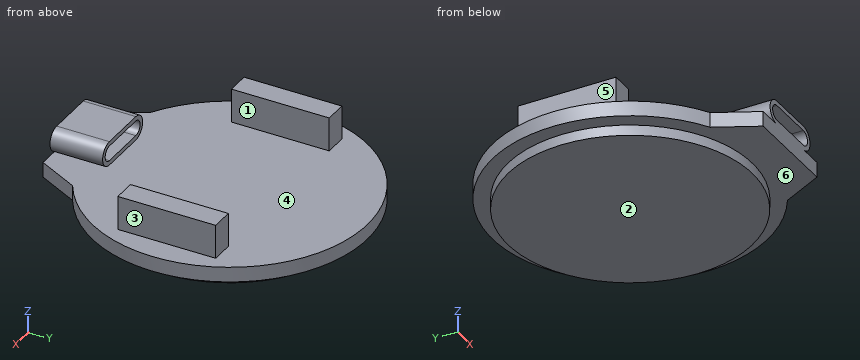
from build123d import *

# Parameters (mm, degrees)
EXTRUDE_1_DEPTH = 2
SKETCH_2_R      = 16.2
EXTRUDE_2_DEPTH = 1.4
SKETCH_3_W      = 3
SKETCH_3_H      = 13
EXTRUDE_3_DEPTH = 4.5
EXTRUDE_4_DEPTH = 7


with BuildPart() as part:
    # 草图1 → 凸台-拉伸1 (new body)
    with BuildSketch(Plane.XY):
        with BuildLine():
            Line((-6.405, -21.250170418), (6.405, -21.250170418))
            Line((6.405, -21.250170418), (9.185, -15.770170418))
            ThreePointArc((9.185, -15.770170418), (0, 18.25), (-9.185, -15.770170418))
            Line((-9.185, -15.770170418), (-6.405, -21.250170418))
        make_face()
    extrude(amount=EXTRUDE_1_DEPTH)

    # 草图2 → 凸台-拉伸2 (add)
    with BuildSketch(Plane(origin=(0, 0, 0), x_dir=(-1, 0, 0), z_dir=(0, 0, -1))):
        Circle(SKETCH_2_R)
    extrude(amount=EXTRUDE_2_DEPTH)

    # 草图3 → 凸台-拉伸3 (add)
    with BuildSketch(Plane.XY.offset(2)):
        with Locations((-13.5, 0)):
            Rectangle(SKETCH_3_W, SKETCH_3_H)
        with Locations((13.5, 0)):
            Rectangle(SKETCH_3_W, SKETCH_3_H)
    extrude(amount=EXTRUDE_3_DEPTH)

    # 草图4 → 凸台-拉伸4 (add)
    with BuildSketch(Plane.XZ.offset(21.250170418)):
        with BuildLine():
            Line((-3.15, 5.2), (3.15, 5.2))
            ThreePointArc((3.15, 5.2), (4.75, 3.6), (3.15, 2))
            Line((3.15, 2), (-3.15, 2))
            ThreePointArc((-3.15, 2), (-4.75, 3.6), (-3.15, 5.2))
        make_face()
        with BuildLine():
            Line((-3.15, 4.6), (3.15, 4.6))
            ThreePointArc((3.15, 4.6), (4.15, 3.6), (3.15, 2.6))
            Line((3.15, 2.6), (-3.15, 2.6))
            ThreePointArc((-3.15, 2.6), (-4.15, 3.6), (-3.15, 4.6))
        make_face(mode=Mode.SUBTRACT)
    extrude(amount=-EXTRUDE_4_DEPTH)


solid = part.part
The listing builds one solid part. Answer for the finished solid, in the listing's coordinates (mm). Face numbers are marked on the shaded views. A direction names the side the tool comes from. Coordinates: 2 decimals unless noted, no trailing zeros. Write each loop counter-clockwise with the first axis right and the second up, starting at its lowest first coordinate (ties: lowest second). Pieces come first, ordered by that corner, then holes. Notation, with made-up numbers: (-31, 79.5) -> (9, 79.5) arc R30 ccw to (9, 114.5) -> close; hole circle Ø11 at (-9, 67.5). An arc over 180 degrees is marked (long way). One line per question, with ' | ' between items.
1. Section A-A (x = 0) is taken. Determine the outline of the cut face in (y, z).
Verdict:
outline: (-21.25, 0) -> (-16.2, 0) -> (-16.2, -1.4) -> (16.2, -1.4) -> (16.2, 0) -> (18.25, 0) -> (18.25, 2) -> (-14.25, 2) -> (-14.25, 2.6) -> (-21.25, 2.6) -> close; (-21.25, 4.6) -> (-14.25, 4.6) -> (-14.25, 5.2) -> (-21.25, 5.2) -> close
2. Section C-C (z = 3.6) is taken. Determine the outline of the cut face in (x, y), and give its area (3 significant figures).
Verdict:
outline: (-15, -6.5) -> (-12, -6.5) -> (-12, 6.5) -> (-15, 6.5) -> close; (-4.75, -21.25) -> (-4.15, -21.25) -> (-4.15, -14.25) -> (-4.75, -14.25) -> close; (4.15, -21.25) -> (4.75, -21.25) -> (4.75, -14.25) -> (4.15, -14.25) -> close; (12, -6.5) -> (15, -6.5) -> (15, 6.5) -> (12, 6.5) -> close | area: 86.4 mm^2
3. Straight lines are drawn through the part: line 1 (X direction, y = -0.5, z = 4.75); line 2 (Z direction, x = 2, y = -0.5); line 3 (Z direction, x = 5, y = 16.5). For each, find the intervals that lie inside material, in ascending order.
Verdict:
line 1: x = -15 to -12, 12 to 15 | line 2: z = -1.4 to 2 | line 3: z = 0 to 2
4. For a pull along X with two mould halves and no side action, classify the marked faces 4, 5 and 6 as released by +X, released by -X, zero draft, split by the parting line, or undercut.
Verdict:
face 4: undercut | face 5: released by -X | face 6: zero draft
5. Which of the six approach directions +Z, -Z, +X, -X, +Y, -Y give full straight-line access (tool end or side, diameter ignored) to the marked faces 1, 2 and 3?
Verdict:
face 1: +Z, +Y, -Y | face 2: -Z, +X, -X, +Y, -Y | face 3: +Z, +X, +Y, -Y
6. Section D-D (y = 0) is taken. Determine the outline of the cut face in (x, z), and give its area (3 significant figures).
Verdict:
outline: (-18.25, 0) -> (-16.2, 0) -> (-16.2, -1.4) -> (16.2, -1.4) -> (16.2, 0) -> (18.25, 0) -> (18.25, 2) -> (15, 2) -> (15, 6.5) -> (12, 6.5) -> (12, 2) -> (-12, 2) -> (-12, 6.5) -> (-15, 6.5) -> (-15, 2) -> (-18.25, 2) -> close | area: 145 mm^2
7. Section B-B (z = 5.75) is taken. Determine the outline of the cut face in (x, y).
Verdict:
outline: (-15, -6.5) -> (-12, -6.5) -> (-12, 6.5) -> (-15, 6.5) -> close; (12, -6.5) -> (15, -6.5) -> (15, 6.5) -> (12, 6.5) -> close
8. Given pin 1 Ø1.3 at (y, z) = (-1.5, 5) entering from +X; pin 2 Ø0.9 at (x, z) = (-14, 3.5) entering from +Y; pin 3 Ø18.5 at (x, y) = (1.5, -3.5) entering from +Z, each flat-ended and moving along its own axis, determine where each tip first touches the part or whether it passes through.
Verdict:
pin 1: stops at x = 15 | pin 2: stops at y = 6.5 | pin 3: stops at z = 2
